Autodesk Inventor part; units mm, degrees
ref_plane "YZ Plane" through (0, 0, 0) normal (1, 0, 0) x (0, 1, 0)
ref_plane "XZ Plane" through (0, 0, 0) normal (0, 1, 0) x (-1, 0, 0)
ref_plane "XY Plane" through (0, 0, 0) normal (0, 0, 1) x (1, 0, 0)
sketch "Boceto1" plane through (0, 0, 0) normal (1, 0, 0) x (0, 1, 0)
  line L0 (27.5, -100) -> (-27.5, -100)
  line L1 (-27.5, -100) -> (-27.5, 100)
  line L2 (-27.5, 100) -> (27.5, 100)
  line L3 (27.5, 100) -> (27.5, -100)
  line L4 (27.5, -100) -> (-27.5, 100) construction
  line L5 (-27.5, -100) -> (27.5, 100) construction
  point P0 (0, 0)
  dimension "alto" = 55
  dimension "ancho" = 200
extrude "Extrusión1" add sketch "Boceto1" along normal blind 18
sketch "Boceto2" plane through (0, 27.5, 100) normal (0, 1, 0) x (1, 0, 0)
  circle A0 centre (9, 66.6667) radius 4.5
  circle A1 centre (9, 133.3333) radius 4.5
  line L0 (0, 0) -> (18, 0)
  line L1 (0, 200) -> (18, 200)
  line L2 (18, 200) -> (18, 0)
  point P0 (0, 100)
  dimension "d4" = 9
  dimension "d5" = 9
  dimension "alto1" = 66.6667
  dimension "d7" = 66.6667
  dimension "d8" = 9
  dimension "d9" = 9
extrude "Extrusión2" cut sketch "Boceto2" against normal blind 6
sketch "Boceto3" plane through (18, 0, 0) normal (1, 0, 0) x (0, 0, -1)
  circle A0 centre (0, -88.1077) radius 80
  line L0 (-100, 27.5) -> (-100, -27.5)
  point P0 (0, 0)
  dimension "radio" = 160
  dimension "d14" = 100
extrude "Extrusión3" cut sketch "Boceto3" against normal blind 18
equation "\"d4\" = 0.5 * grosor"
equation "\"d5\" = d4"
equation "\"d7\" = alto1"
equation "\"d8\" = d9"
equation "\"d9\" = 0.5 * grosor"
equation "\"d10\" = 0.333333 * grosor"
equation "\"d14\" = 0.5 * ancho"
equation "\"d15\" = grosor"
properties part number "soporte"
Design review of the part built by this model. Coordinates are the model's own, in mm. A direction names the side the tool comes from. Coordinates: 2 decimals unless noted, no trailing zeros. Loops run counter-clockwise (first coordinate to the right, second up) from the corner with the lowest first, then second, coordinate; pieces in that order, holes last.
Q1. For pin 1 (8 mm diameter, centred on x = 9, z = -33.33, fed in from +Y); pin 2 (10.5 mm diameter, centred on x = 9, z = 33.33, fed in from -Y) (3 decimals), all flat-tipped, find the tip position at first contact; note any pin that passes through.
Reported:
pin 1: stops at y = 21.5
pin 2: stops at y = -18.025
Q2. To check wall thickness, follow line 1 (Z direction, x = 9, y = 24.8); line 2 (Z direction, x = 8, y = -16.5); line 3 (Y direction, x = 15.5, z = 6.5). State the ranges of each line that lie inside material, in increasing order.
Reported:
line 1: z = -100 to -37.83, -28.83 to 28.83, 37.83 to 100
line 2: z = -100 to -35.67, 35.67 to 100
line 3: y = -8.37 to 27.5
Q3. The part is to be moulded in two halves that separate along Z. For faces 1 (the face through (9, 0, -100)), 2 (the face through (9, 0, 100)), 3 (the face through (9.13, -8.11, -0.8)), say which applies: +Z half, -Z half, draft (parallel to the pull), parting line (faces both ways), or undercut.
Reported:
face 1: -Z half
face 2: +Z half
face 3: undercut
Q4. We need section A-A on y = -11. State the section outline as (x, z) points, and give its area (3 significant figures).
Reported:
outline: (0, -100) - (18, -100) - (18, -21.32) - (0, -21.32) - close; (0, 21.32) - (18, 21.32) - (18, 100) - (0, 100) - close
area: 2,830 mm2
Q5. Tool access review of faces 4 (the face through (11.419, 24.542, -37.128)), 5 (the face through (9, -27.5, 76)): name each direction out of +Z, -Z, +X, -X, +Y, -Y from which nothing blocks a thin tool from reaching the whole face with its end or side.
Reported:
face 4: +Y
face 5: +Z, -Z, +X, -X, -Y
Q6. We need section D-D on z = -3. State the section outline as (x, y) points, and give its area (3 significant figures).
Reported:
outline: (0, -8.16) - (18, -8.16) - (18, 27.5) - (0, 27.5) - close
area: 642 mm2
Q7. We need section C-C on y = 24.5. State the section outline as (x, z) points, and give its area (3 significant figures).
Reported:
outline: (0, -100) - (18, -100) - (18, 100) - (0, 100) - close; hole circle Ø9 at (9, -33.33); hole circle Ø9 at (9, 33.33)
area: 3,470 mm2
Q8. We need section B-B on x = 15.75. State the section outline as (y, z) points.
Reported:
outline: (-27.5, -100) - (27.5, -100) - (27.5, 100) - (-27.5, 100) - (-27.5, 52.22) arc R80 cw to (-27.5, -52.22) - close
